Verification items for the finished model (mm, model axes). A direction names the side the tool comes from. Coordinates: 2 decimals unless noted, no trailing zeros. Order: outer loops, then holes, each group sorted by start corner. A loop starts at its lowest first (then second) coordinate and runs counter-clockwise, first axis right, second up. Notation, with made-up numbers: (-22, 89) -> (-8, 89) arc R8 ccw to (-8, 100) -> close; hole circle Ø9 at (-39, -34). An arc over 180 degrees is marked (long way). Write each question's results on one line, items separated by ' | '. Start each with the question number.
(1) Draft check along X on faces 1 (the flat face through (0, 4, 74)), 2 (the cylindrical face through (-0.08, 2.25, 73.95)), 3 (the cylindrical face through (4.443, 8.811, 73.95)), 4 (the flat face through (1.5, 3.8, 0)). Enter one of: +X half, -X half, draft (parallel to the pull), parting line (faces both ways), or undercut.
(2) Cross-section at A-A on y = 0. Enter the section's corners in (x, z), and give its area (3 significant figures).
(3) Cross-section at C-C on y = 9.25. Enter the section's corners in (x, z).
(4) Thickness scan on probe 1 along Y at (x, z) = (0, 46); probe 2 along Y at (x, z) = (-1.75, 95); probe 3 along X at (y, z) = (0, 114). Record the ranges inside material, lowest first. Write a range as [from, to].
(5) Set-up check for faces 5 (the flat face through (-5, 5.383, 74)), 6 (the flat face through (7, 4, 74)): record each of +Z, -Z, +X, -X, +Y, -Y from which the full face is reachable in a straight line by a thin tool's end or side.
(6) Cross-section at B-B on z = 26.5. Enter the section's corners in (x, y), and give its area (3 significant figures).
(7) Go/stop test with flat-tipped pins: pin 1 (2 mm diameter, centred on y = 0, z = 41, fed in from -X); pin 2 (1.1 mm diameter, centred on x = -6, z = 68, fed in from +Y); pin 3 (1.5 mm diameter, centred on y = 7, z = 131, fed in from +X). Record where each tip stops, or that it passes through.
```python
from build123d import *

# Parameters (mm, degrees)
F1_DEPTH = 150


with BuildPart() as f1:
    # F0 (on Top) → F1 (new body)
    with BuildSketch(Plane.XY):
        Polygon((7, 2.5), (7, 4), (4.5, 4), (-4.5, 4), (-7, 4), (-7, 2.5), align=None)
        Polygon((4.5, 4), (7, 4), (7, 5.382979), (3.339543, 5.382979), align=None)
        with BuildLine():
            Line((3, -2.015564), (7, 2.5))
            Line((7, 2.5), (-7, 2.5))
            Line((-7, 2.5), (-3, -2.015564))
            Line((-3, -2.015564), (-1, -2.015564))
            ThreePointArc((-1, -2.015564), (0, 2.25), (1, -2.015564))
            Line((1, -2.015564), (3, -2.015564))
        make_face()
        with BuildLine():
            Line((3.339543, 5.382979), (7, 5.382979))
            ThreePointArc((7, 5.382979), (6.546372, 9.016241), (5.21334, 12.426431))
            ThreePointArc((5.21334, 12.426431), (4.929027, 12.548792), (4.743648, 12.300918))
            ThreePointArc((4.743648, 12.300918), (4.433508, 8.762404), (3.339543, 5.382979))
        make_face()
        Polygon((-7, 4), (-4.5, 4), (-3.339543, 5.382979), (-7, 5.382979), align=None)
    extrude(amount=F1_DEPTH)


solid = f1.part
```
Results are:
1) face 1: undercut | face 2: undercut | face 3: -X half | face 4: draft
2) outline: (-4.79, 0) -> (-2.25, 0) -> (-2.25, 150) -> (-4.79, 150) -> close; (2.25, 0) -> (4.79, 0) -> (4.79, 150) -> (2.25, 150) -> close | area: 761 mm2
3) outline: (4.52, 0) -> (6.49, 0) -> (6.49, 150) -> (4.52, 150) -> close
4) probe 1: y = [2.25, 4] | probe 2: y = [-2.02, -1.41], [1.41, 4] | probe 3: x = [-4.79, -2.25], [2.25, 4.79]
5) face 5: +Z, -Z, -X, +Y | face 6: +Z, -Z, +X, +Y, -Y
6) outline: (-7, 2.5) -> (-3, -2.02) -> (-1, -2.02) arc R2.25 cw (long way) to (1, -2.02) -> (3, -2.02) -> (7, 2.5) -> (7, 5.38) arc R14.78 ccw to (5.21, 12.43) arc R0.25 ccw to (4.74, 12.3) arc R15.78 cw to (3.34, 5.38) -> (4.5, 4) -> (-4.5, 4) -> (-3.34, 5.38) -> (-7, 5.38) -> close | area: 73.9 mm2
7) pin 1: stops at x = -5.67 | pin 2: stops at y = 5.38 | pin 3: stops at x = 6.97
